Part model, mm, in its own coordinate system. A direction names the side the tool comes from. Round coordinates to 2 decimals unless told otherwise and drop trailing zeros. Order: outer loops, then holes, each group sorted by start corner. A loop starts at its lowest first (then second) coordinate and runs counter-clockwise, first axis right, second up. Notation, with made-up numbers: (53, 18) - (67, 18) arc R27 ccw to (67, 40) - close; hole circle Ø8 at (-28.5, 2). An arc over 180 degrees is marked (long way). Return JSON: item names as keys, results as strings. Group by question number.
Item 1: Probe probe 1 along X at (y, z) = (0.7, -2.2); probe 2 along X at (y, z) = (2.5, -13.25); probe 3 along X at (y, z) = (7.5, -8). List the from-to ranges inside material, lowest first.
Item 2: Saw through at A-A on z = -2.2. List the corners of the cut face in (x, y), and give its area (3 significant figures).
Item 3: Two-plate mould, pull along X, no slides. Class faces 1 (the face through (4.2, 5, -10)), 2 (the face through (4.347, 0.811, -1.6)), 3 (the face through (10, 27.5, -10)): released by +X, released by -X, zero draft, split by the parting line, or undercut.
Item 4: Drop flat-ended pins along their axis: pin 1 (1.6 mm diameter, centred on y = 3.5, z = -12.5, fed in from +X); pin 2 (3 mm diameter, centred on y = 4, z = -9, fed in from -X); pin 3 (5 mm diameter, centred on x = 13.5, y = 22, fed in from +Z). Give the stop position or say it passes through.
Item 5: Saw through at B-B on x = 19. List the corners of the cut face in (y, z), and give its area (3 significant figures).
Item 6: Tool access for faces 4 (the face through (16.2, 5, -10)), 5 (the face through (26.4, 1, -9)), 6 (the face through (27, 5.4, -10)), 7 (the face through (10, 17.5, -12)): list every direction of +Z, -Z, +X, -X, +Y, -Y with a clear straight run to the whole face (end or side of a thin tool).
Item 7: Saw through at D-D on x = 15. List the corners of the cut face in (y, z), and give its area (3 significant figures).
Item 8: Saw through at C-C on z = -15. List the corners of the cut face in (x, y), and give its area (3 significant figures).
```python
from build123d import *

# Parameters (mm, degrees)
SKETCH2_W           = 26.4
SKETCH2_H           = 19
BOSS_EXTRUDE1_DEPTH = 1.6
SKETCH3_R           = 1.3
CUT_EXTRUDE1_DEPTH  = 33.56562605
SKETCH4_W           = 12
SKETCH4_H           = 12
BOSS_EXTRUDE2_DEPTH = 6.1
SKETCH5_R           = 3.4
BOSS_EXTRUDE3_DEPTH = 6.8
SKETCH6_R           = 3
BOSS_EXTRUDE4_DEPTH = 3
BOSS_EXTRUDE5_DEPTH = 10
SKETCH8_W           = 3
SKETCH8_H           = 12
SKETCH8_W_2         = 5
BOSS_EXTRUDE6_DEPTH = 3.8
SKETCH9_W           = 5.6
SKETCH9_H           = 3.2
CUT_EXTRUDE2_DEPTH  = 45.286002303


with BuildPart() as part:
    # Sketch2 → Boss-Extrude1 (new body)
    with BuildSketch(Plane(origin=(0, 0, 0), x_dir=(1, 0, 0), z_dir=(0, 1, 0))):
        with Locations((13.2, 9.5)):
            Rectangle(SKETCH2_W, SKETCH2_H)
    extrude(amount=BOSS_EXTRUDE1_DEPTH)

    # Sketch3 → Cut-Extrude1 (cut, through all)
    with BuildSketch(Plane(origin=(0, 1.6, 0), x_dir=(1, 0, 0), z_dir=(0, 1, 0))):
        with Locations(Location((5.5, 2.2, 0), (0, 0, 270))):
            Circle(SKETCH3_R)
        with Locations(Location((19, 2.2, 0), (0, 0, 270))):
            Circle(SKETCH3_R)
    extrude(amount=-CUT_EXTRUDE1_DEPTH, mode=Mode.SUBTRACT)

    # Sketch4 → Boss-Extrude2 (add)
    with BuildSketch(Plane(origin=(0, 1.6, 0), x_dir=(1, 0, 0), z_dir=(0, 1, 0))):
        with Locations((10.2, 10.2)):
            Rectangle(SKETCH4_W, SKETCH4_H)
    extrude(amount=BOSS_EXTRUDE2_DEPTH)

    # Sketch5 → Boss-Extrude3 (add)
    with BuildSketch(Plane(origin=(0, 7.7, 0), x_dir=(1, 0, 0), z_dir=(0, 1, 0))):
        with Locations(Location((10.2, 10.2, 0), (0, 0, 270))):
            Circle(SKETCH5_R)
    extrude(amount=BOSS_EXTRUDE3_DEPTH)

    # Sketch6 → Boss-Extrude4 (add)
    with BuildSketch(Plane(origin=(0, 14.5, 0), x_dir=(1, 0, 0), z_dir=(0, 1, 0))):
        with Locations(Location((10.2, 10.2, 0), (0, 0, 270))):
            Circle(SKETCH6_R)
    extrude(amount=BOSS_EXTRUDE4_DEPTH)

    # Sketch7 → Boss-Extrude5 (add)
    with BuildSketch(Plane(origin=(0, 17.5, 0), x_dir=(1, 0, 0), z_dir=(0, 1, 0))):
        with BuildLine():
            ThreePointArc((13.2, 10.2), (13.097777479, 10.976457135), (12.798076211, 11.7))
            Line((12.798076211, 11.7), (12.798076211, 8.7))
            ThreePointArc((12.798076211, 8.7), (13.097777479, 9.423542865), (13.2, 10.2))
        make_face()
        with BuildLine():
            Line((7.601923789, 8.7), (7.601923789, 11.7))
            ThreePointArc((7.601923789, 11.7), (7.2, 10.2), (7.601923789, 8.7))
        make_face()
        with BuildLine():
            Line((12.798076211, 11.7), (7.601923789, 11.7))
            Line((7.601923789, 11.7), (7.601923789, 8.7))
            ThreePointArc((7.601923789, 8.7), (8.7, 7.601923789), (10.2, 7.2))
            ThreePointArc((10.2, 7.2), (11.7, 7.601923789), (12.798076211, 8.7))
            Line((12.798076211, 8.7), (12.798076211, 11.7))
        make_face()
    extrude(amount=BOSS_EXTRUDE5_DEPTH)

    # Sketch8 → Boss-Extrude6 (add)
    with BuildSketch(Plane(origin=(0, 1.6, 0), x_dir=(1, 0, 0), z_dir=(0, 1, 0))):
        with Locations((24.9, 10.2)):
            Rectangle(SKETCH8_W, SKETCH8_H)
        with Locations((28.9, 10.2)):
            Rectangle(SKETCH8_W_2, SKETCH8_H)
    extrude(amount=BOSS_EXTRUDE6_DEPTH)

    # Sketch9 → Cut-Extrude2 (cut, through all)
    with BuildSketch(Plane.XY.offset(-4.2)):
        with Locations((28.6, 3.2)):
            Rectangle(SKETCH9_W, SKETCH9_H)
    extrude(amount=-CUT_EXTRUDE2_DEPTH, mode=Mode.SUBTRACT)


solid = part.part
```
Filled in:
{
 "1": {"probe 1": "x = 0 to 4.2, 6.8 to 17.7, 20.3 to 26.4", "probe 2": "x = 4.2 to 16.2, 23.4 to 25.8", "probe 3": "x = 4.2 to 16.2"},
 "2": {"outline": "(0, 0) - (4.2, 0) - (4.2, 1.6) - (0, 1.6) - close; (6.8, 0) - (17.7, 0) - (17.7, 1.6) - (6.8, 1.6) - close; (20.3, 0) - (26.4, 0) - (26.4, 1.6) - (20.3, 1.6) - close", "area": "33.9 mm^2"},
 "3": {"face 1": "released by -X", "face 2": "undercut", "face 3": "zero draft"},
 "4": {"pin 1": "stops at x = 25.8", "pin 2": "stops at x = 4.2", "pin 3": "stops at z = -7.31"},
 "5": {"outline": "(0, -19) - (1.6, -19) - (1.6, -3.5) - (0, -3.5) - close; (0, -0.9) - (1.6, -0.9) - (1.6, 0) - (0, 0) - close", "area": "26.2 mm^2"},
 "6": {"face 4": "+Z, -Z, +Y", "face 5": "+Z, -Z, +X, -Y", "face 6": "+Z, -Z, +X, +Y", "face 7": "-Z, +X, -X, +Y"},
 "7": {"outline": "(0, -19) - (1.6, -19) - (1.6, -16.2) - (7.7, -16.2) - (7.7, -4.2) - (1.6, -4.2) - (1.6, 0) - (0, 0) - close", "area": "104 mm^2"},
 "8": {"outline": "(0, 0) - (26.4, 0) - (26.4, 1.6) - (25.8, 1.6) - (25.8, 4.8) - (31.4, 4.8) - (31.4, 5.4) - (23.4, 5.4) - (23.4, 1.6) - (16.2, 1.6) - (16.2, 7.7) - (4.2, 7.7) - (4.2, 1.6) - (0, 1.6) - close", "area": "128 mm^2"}
}
